from build123d import *

# Parameters (mm, degrees)
SKETCH_1_R          = 13
SKETCH_1_R_2        = 11
EXTRUDE_1_DEPTH     = 460
SKETCH_2_R          = 2
SKETCH_2_R_2        = 2.5
CUT_EXTRUDE_1_DEPTH = 14
SKETCH_4_R          = 1.5
CUT_EXTRUDE_2_DEPTH = 14.0000001


with BuildPart() as part:
    # 草图1 → 凸台-拉伸1 (new body)
    with BuildSketch(Plane(origin=(0, 0, 0), x_dir=(0, 0, -1), z_dir=(1, 0, 0))):
        Circle(SKETCH_1_R)
        Circle(SKETCH_1_R_2, mode=Mode.SUBTRACT)
    extrude(amount=EXTRUDE_1_DEPTH)

    # 草图2 → 切除-拉伸1 (cut, through all)
    with BuildSketch(Plane.XY):
        with Locations((21, 0)):
            Circle(SKETCH_2_R)
        with Locations((445, 0)):
            Circle(SKETCH_2_R_2)
    extrude(amount=-CUT_EXTRUDE_1_DEPTH, mode=Mode.SUBTRACT)

    # 草图4 → 切除-拉伸2 (cut, through all)
    with BuildSketch(Plane(origin=(0, 0, 0), x_dir=(1, 0, 0), z_dir=(0, 1, 0))):
        with Locations((12.5, 0)):
            Circle(SKETCH_4_R)
        with Locations((441.5, 0)):
            Circle(SKETCH_4_R)
    extrude(amount=-CUT_EXTRUDE_2_DEPTH, mode=Mode.SUBTRACT)


solid = part.part
CAD build for the part. Positions are in the model's coordinates, mm. Round coordinates to 2 decimals unless told otherwise and drop trailing zeros. Write each loop counter-clockwise with the first axis right and the second up, starting at its lowest first coordinate (ties: lowest second). Pieces come first, ordered by that corner, then holes. Notation, with made-up numbers: M 70,56.5 L 87,56.5 A18 ccw 87,82.5 Z; hole C 24.25,32.5 d4. An arc over 180 degrees is marked long. Put each result on its own line as item: value. Start each with the question number.
1) Pull direction Y, two halves, no side cores. Call faces 1 (the flat face through (0, 3, 11)), 2 (the cylindrical face through (226.78, -7.91, 10.316)), 3 (the cylindrical face through (226.78, -10.74, 2.38)): pulls with the +Y half, pulls with the -Y half, needs draft (parallel to the pull), parting line crosses it, or undercut.
2) Saw through at B-B, the plane x = 417.5. Write the cut outline in (y, z).
3) Saw through at A-A, the plane z = -5.5. Write the cut outline in (x, y), and give its area (3 significant figures).
4) Drill centre lines: probe 1 along X at (y, z) = (-12.05, 0); probe 2 along X at (y, z) = (0, -12.15); probe 3 along Y at (x, z) = (122.5, 0). Where is each one in solid material? Low to high. Write a range as [from, to].
5) Pin check, flat tips, straight feed: pin 1 Ø12 at (x, z) = (350.5, 3) entering from +Y; pin 2 Ø3 at (x, y) = (21, 0) entering from -Z; pin 3 Ø1.8 at (x, z) = (12.5, 0) entering from -Y; pin 4 Ø4 at (x, y) = (170, -8.5) entering from +Z. Stop position of each tip, or through.
Resolved:
1. face 1: needs draft
1. face 2: parting line crosses it
1. face 3: undercut
2. outline: C 0,0 d26; hole C 0,0 d22
3. outline: M 0,-11.78 L 460,-11.78 L 460,-9.53 L 0,-9.53 Z; M 0,9.53 L 460,9.53 L 460,11.78 L 0,11.78 Z
3. area: 2,070 mm²
4. probe 1: [0, 11], [14, 440], [443, 460]
4. probe 2: [0, 19], [23, 442.5], [447.5, 460]
4. probe 3: [-13, -11], [11, 13]
5. pin 1: y = 13
5. pin 2: z = 10.9
5. pin 3: y = 10.96
5. pin 4: z = 11.26
